Autodesk Inventor part; units mm, degrees
ref_plane "YZ Plane" through (0, 0, 0) normal (1, 0, 0) x (0, 1, 0)
ref_plane "XZ Plane" through (0, 0, 0) normal (0, 1, 0) x (-1, 0, 0)
ref_plane "XY Plane" through (0, 0, 0) normal (0, 0, 1) x (1, 0, 0)
sketch "Sketch1" plane through (0, 0, 0) normal (0, 0, 1) x (1, 0, 0)
  line L0 (-5.91, 5.4476) -> (654.49, 5.4476)
  line L1 (654.49, 5.4476) -> (654.49, -19.9524)
  line L2 (654.49, -19.9524) -> (-5.91, -19.9524)
  line L3 (-5.91, -19.9524) -> (-5.91, 5.4476)
  point P0 (0, 0)
  dimension "d0" = 660.4
  dimension "d1" = 25.4
extrude "Extrusion1" add sketch "Sketch1" along normal blind 25.4
sketch "Sketch2" plane through (0, 0, 25.4) normal (0, 0, 1) x (1, 0, 0)
  circle A0 centre (6.79, -7.2524) radius 1.9685
  line L0 (-5.91, 5.4476) -> (-5.91, -19.9524)
  line L1 (-5.91, -19.9524) -> (654.49, -19.9524)
  circle A1 centre (32.19, -7.2524) radius 1.9685
  circle A2 centre (57.59, -7.2524) radius 1.9685
  circle A3 centre (82.99, -7.2524) radius 1.9685
  circle A4 centre (108.39, -7.2524) radius 1.9685
  circle A5 centre (133.79, -7.2524) radius 1.9685
  circle A6 centre (159.19, -7.2524) radius 1.9685
  circle A7 centre (184.59, -7.2524) radius 1.9685
  circle A8 centre (209.99, -7.2524) radius 1.9685
  circle A9 centre (235.39, -7.2524) radius 1.9685
  circle A10 centre (260.79, -7.2524) radius 1.9685
  circle A11 centre (286.19, -7.2524) radius 1.9685
  circle A12 centre (311.59, -7.2524) radius 1.9685
  circle A13 centre (336.99, -7.2524) radius 1.9685
  circle A14 centre (362.39, -7.2524) radius 1.9685
  circle A15 centre (387.79, -7.2524) radius 1.9685
  circle A16 centre (413.19, -7.2524) radius 1.9685
  circle A17 centre (438.59, -7.2524) radius 1.9685
  circle A18 centre (463.99, -7.2524) radius 1.9685
  circle A19 centre (489.39, -7.2524) radius 1.9685
  circle A20 centre (514.79, -7.2524) radius 1.9685
  circle A21 centre (540.19, -7.2524) radius 1.9685
  circle A22 centre (565.59, -7.2524) radius 1.9685
  circle A23 centre (590.99, -7.2524) radius 1.9685
  circle A24 centre (616.39, -7.2524) radius 1.9685
  circle A25 centre (641.79, -7.2524) radius 1.9685
  point P0 (0, 0)
  dimension "d4" = 3.937
  dimension "d5" = 12.7
  dimension "d6" = 12.7
  dimension "d9" = 25.4
  dimension "d16" = 25.4
extrude "Extrusion2" cut sketch "Sketch2" against normal blind 25.4
sketch "Sketch3" plane through (-5.91, -19.9524, 0) normal (-1, 0, 0) x (0, 0, 1)
  line L0 (3.175, 22.225) -> (22.225, 22.225)
  line L1 (22.225, 22.225) -> (22.225, 3.175)
  line L2 (22.225, 3.175) -> (3.175, 3.175)
  line L3 (3.175, 3.175) -> (3.175, 22.225)
  line L4 (0, 25.4) -> (25.4, 25.4)
  line L5 (0, 0) -> (0, 25.4)
  line L6 (0, 0) -> (25.4, 0)
  line L7 (25.4, 25.4) -> (25.4, 0)
  point P0 (0, 19.9524)
  dimension "d23" = 3.175
  dimension "d24" = 3.175
  dimension "d25" = 3.175
  dimension "d26" = 3.175
sketch "Sketch4" plane through (-5.91, 5.4476, 0) normal (0, 1, 0) x (1, 0, 0)
  circle A0 centre (12.7, -12.7) radius 1.9685
  line L0 (0, 0) -> (0, -25.4)
  line L1 (660.4, -25.4) -> (0, -25.4)
  circle A1 centre (38.1, -12.7) radius 1.9685
  circle A2 centre (63.5, -12.7) radius 1.9685
  circle A3 centre (88.9, -12.7) radius 1.9685
  circle A4 centre (114.3, -12.7) radius 1.9685
  circle A5 centre (139.7, -12.7) radius 1.9685
  circle A6 centre (165.1, -12.7) radius 1.9685
  circle A7 centre (190.5, -12.7) radius 1.9685
  circle A8 centre (215.9, -12.7) radius 1.9685
  circle A9 centre (241.3, -12.7) radius 1.9685
  circle A10 centre (266.7, -12.7) radius 1.9685
  circle A11 centre (292.1, -12.7) radius 1.9685
  circle A12 centre (317.5, -12.7) radius 1.9685
  circle A13 centre (342.9, -12.7) radius 1.9685
  circle A14 centre (368.3, -12.7) radius 1.9685
  circle A15 centre (393.7, -12.7) radius 1.9685
  circle A16 centre (419.1, -12.7) radius 1.9685
  circle A17 centre (444.5, -12.7) radius 1.9685
  circle A18 centre (469.9, -12.7) radius 1.9685
  circle A19 centre (495.3, -12.7) radius 1.9685
  circle A20 centre (520.7, -12.7) radius 1.9685
  circle A21 centre (546.1, -12.7) radius 1.9685
  circle A22 centre (571.5, -12.7) radius 1.9685
  circle A23 centre (596.9, -12.7) radius 1.9685
  circle A24 centre (622.3, -12.7) radius 1.9685
  circle A25 centre (647.7, -12.7) radius 1.9685
  point P0 (5.91, 0)
  dimension "d27" = 3.937
  dimension "d28" = 12.7
  dimension "d29" = 12.7
  dimension "d32" = 25.4
extrude "Extrusion3" cut sketch "Sketch4" against normal blind 25.4
extrude "Extrusion4" cut sketch "Sketch3" against normal blind 660.4 contours L0 L1 L2 L3
sketch "Sketch5" plane through (654.49, -19.9524, 0) normal (1, 0, 0) x (0, 0, -1)
  line L0 (-25.4, 25.4) -> (-25.4, 0)
  line L1 (-25.4, 25.4) -> (0, 25.4)
  line L2 (0, 25.4) -> (0, 0)
  line L3 (0, 0) -> (-25.4, 0)
  line L4 (-25.4, 0) -> (-25.4, 25.4)
  point P0 (0, 19.9524)
extrude "Extrusion5" cut sketch "Sketch5" against normal blind 393.7
properties part number "real numbah 9"
Part model, mm, in its own coordinate system. A direction names the side the tool comes from. Give positions to 0.01 mm unless a question says otherwise; leave off trailing zeros. Order: outer loops, then holes, each group sorted by start corner. A loop starts at its lowest first (then second) coordinate and runs counter-clockwise, first axis right, second up. Notation, with made-up numbers: M 78.25,-37 L 101.25,-37 A19 cw 101.25,-3 Z; hole C 38,15.25 d11. An arc over 180 degrees is marked long. Use a Markdown table: item, result. Add a question column.
(1) Probe line 1 along Y through (x, z) = (235.39, 1.7); line 2 along Y through (x, z) = (243, 11); line 3 along Z through (x, y) = (210, -13.75) (3 decimals). List the from-to ranges inside material, lowest first. Write a range as [from, to].
(2) Drop flat-ended pins along their axis: P1, Ø2, axis at x = 82, y = -5, coming from the -Z side; P2, Ø3, axis at x = 6.79, y = -7.25, coming from the -Z side. Give the stop position or say it passes through.
(3) Saw through at B-B, the plane y = -13.5. Give the cut face in (x, z) (3 decimals), and give its area (3 significant figures).
(4) Saw through at A-A, the plane z = 7.75. Give the cut face in (x, y).
(5) 3-axis set-ups, long thin cutter, end or side, ignore diameter. For faces 1 (the face through (126, -16.777, 13)), 2 (the face through (129, -19.952, 13)): which of +Z, -Z, +X, -X, +Y, -Y reach the whole face in a straight line?
(6) Mould opens along Z. For faces 3 (the face through (126, -7, 0)), 4 (the face through (126, -7, 22.225)), 5 (the face through (-5.91, -19, 13)), 6 (the face through (126, -7, 3.175)) say: +Z half, -Z half, draft (parallel to the pull), parting line (faces both ways), or undercut.
(7) Saw through at C-C, the plane x = 146.5. Give the cut face in (y, z) (3 decimals).
Answer key:
| question | item | result |
|---|---|---|
| 1 | line 1 | [-19.95, -9.22], [-5.28, 5.45] |
| 1 | line 2 | [-19.95, -16.78], [2.27, 5.45] |
| 1 | line 3 | [0, 3.175], [22.225, 25.4] |
| 2 | P1 | z = 0 |
| 2 | P2 | through |
| 3 | outline | M -5.91,0 L 260.79,0 L 260.79,3.175 L -5.91,3.175 Z; M -5.91,22.225 L 260.79,22.225 L 260.79,25.4 L -5.91,25.4 Z |
| 3 | area | 1,690 mm^2 |
| 4 | outline | M -5.91,-19.95 L 260.79,-19.95 L 260.79,-16.78 L -5.91,-16.78 Z; M -5.91,2.27 L 260.79,2.27 L 260.79,5.45 L -5.91,5.45 Z |
| 5 | face 1 | +X, -X |
| 5 | face 2 | +Z, -Z, +X, -X, -Y |
| 6 | face 3 | -Z half |
| 6 | face 4 | undercut |
| 6 | face 5 | draft |
| 6 | face 6 | undercut |
| 7 | outline | M -19.952,0 L 5.448,0 L 5.448,25.4 L -19.952,25.4 Z; hole M -16.777,3.175 L 2.273,3.175 L 2.273,22.225 L -16.777,22.225 Z |
